```python
from build123d import *

# Parameters (mm, degrees)
F0_W     = 60
F0_H     = 20
F1_DEPTH = 5
F3_DEPTH = 2


with BuildPart() as f1:
    # F0 (on Top) → F1 (new body)
    with BuildSketch(Plane.XY):
        Rectangle(F0_W, F0_H)
    extrude(amount=F1_DEPTH)

    # F2 (on face) → F3 (cut)
    with BuildSketch(Plane.XY.offset(5)):
        with BuildLine():
            ThreePointArc((-8.9875, -4.4832849285), (-7.8815819875, -2.3618054535), (-7.5, 0))
            ThreePointArc((-7.5, 0), (-7.8815819875, 2.3618054535), (-8.9875, 4.4832849285))
            ThreePointArc((-8.9875, 4.4832849285), (-9.5314526404, 3.9326755483), (-10, 3.3166247904))
            ThreePointArc((-10, 3.3166247904), (-9.2554373535, 1.7320508076), (-9, 0))
            ThreePointArc((-9, 0), (-9.2554373535, -1.7320508076), (-10, -3.3166247904))
            ThreePointArc((-10, -3.3166247904), (-9.5314526404, -3.9326755483), (-8.9875, -4.4832849285))
        make_face()
        with BuildLine():
            ThreePointArc((-10, 3.3166247904), (-9.5314526404, 3.9326755483), (-8.9875, 4.4832849285))
            ThreePointArc((-8.9875, 4.4832849285), (-9.4660061735, 5.0621055232), (-10, 5.5901699437))
            ThreePointArc((-10, 5.5901699437), (-10.5339938265, 5.0621055232), (-11.0125, 4.4832849285))
            ThreePointArc((-11.0125, 4.4832849285), (-10.4685473596, 3.9326755483), (-10, 3.3166247904))
        make_face()
        with BuildLine():
            ThreePointArc((-10, 5.5901699437), (-9.4660061735, 5.0621055232), (-8.9875, 4.4832849285))
            ThreePointArc((-8.9875, 4.4832849285), (-5, 6), (-1.0125, 4.4832849285))
            ThreePointArc((-1.0125, 4.4832849285), (-0.5339938265, 5.0621055232), (0, 5.5901699437))
            ThreePointArc((0, 5.5901699437), (-5, 7.5), (-10, 5.5901699437))
        make_face()
        with BuildLine():
            ThreePointArc((-1.0125, -4.4832849285), (-5, -6), (-8.9875, -4.4832849285))
            ThreePointArc((-8.9875, -4.4832849285), (-9.4660061735, -5.0621055232), (-10, -5.5901699437))
            ThreePointArc((-10, -5.5901699437), (-5, -7.5), (0, -5.5901699437))
            ThreePointArc((0, -5.5901699437), (-0.5339938265, -5.0621055232), (-1.0125, -4.4832849285))
        make_face()
        with BuildLine():
            ThreePointArc((-10, -5.5901699437), (-9.4660061735, -5.0621055232), (-8.9875, -4.4832849285))
            ThreePointArc((-8.9875, -4.4832849285), (-9.5314526404, -3.9326755483), (-10, -3.3166247904))
            ThreePointArc((-10, -3.3166247904), (-10.4685473596, -3.9326755483), (-11.0125, -4.4832849285))
            ThreePointArc((-11.0125, -4.4832849285), (-10.5339938265, -5.0621055232), (-10, -5.5901699437))
        make_face()
        with BuildLine():
            ThreePointArc((-11.0125, 4.4832849285), (-10.5339938265, 5.0621055232), (-10, 5.5901699437))
            ThreePointArc((-10, 5.5901699437), (-22.5, 0), (-10, -5.5901699437))
            ThreePointArc((-10, -5.5901699437), (-10.5339938265, -5.0621055232), (-11.0125, -4.4832849285))
            ThreePointArc((-11.0125, -4.4832849285), (-21, 0), (-11.0125, 4.4832849285))
        make_face()
        with BuildLine():
            ThreePointArc((0, 5.5901699437), (-0.5339938265, 5.0621055232), (-1.0125, 4.4832849285))
            ThreePointArc((-1.0125, 4.4832849285), (-0.4685473596, 3.9326755483), (0, 3.3166247904))
            ThreePointArc((0, 3.3166247904), (0.4685473596, 3.9326755483), (1.0125, 4.4832849285))
            ThreePointArc((1.0125, 4.4832849285), (0.5339938265, 5.0621055232), (0, 5.5901699437))
        make_face()
        with BuildLine():
            ThreePointArc((0, 3.3166247904), (-0.4685473596, 3.9326755483), (-1.0125, 4.4832849285))
            ThreePointArc((-1.0125, 4.4832849285), (-2.5, 0), (-1.0125, -4.4832849285))
            ThreePointArc((-1.0125, -4.4832849285), (-0.4685473596, -3.9326755483), (0, -3.3166247904))
            ThreePointArc((0, -3.3166247904), (-1, 0), (0, 3.3166247904))
        make_face()
        with BuildLine():
            ThreePointArc((-10, -3.3166247904), (-11, 0), (-10, 3.3166247904))
            ThreePointArc((-10, 3.3166247904), (-10.4685473596, 3.9326755483), (-11.0125, 4.4832849285))
            ThreePointArc((-11.0125, 4.4832849285), (-12.5, 0), (-11.0125, -4.4832849285))
            ThreePointArc((-11.0125, -4.4832849285), (-10.4685473596, -3.9326755483), (-10, -3.3166247904))
        make_face()
        with BuildLine():
            ThreePointArc((0, -3.3166247904), (-0.4685473596, -3.9326755483), (-1.0125, -4.4832849285))
            ThreePointArc((-1.0125, -4.4832849285), (-0.5339938265, -5.0621055232), (0, -5.5901699437))
            ThreePointArc((0, -5.5901699437), (0.5339938265, -5.0621055232), (1.0125, -4.4832849285))
            ThreePointArc((1.0125, -4.4832849285), (0.4685473596, -3.9326755483), (0, -3.3166247904))
        make_face()
        with BuildLine():
            ThreePointArc((10, 5.5901699437), (5, 7.5), (0, 5.5901699437))
            ThreePointArc((0, 5.5901699437), (0.5339938265, 5.0621055232), (1.0125, 4.4832849285))
            ThreePointArc((1.0125, 4.4832849285), (5, 6), (8.9875, 4.4832849285))
            ThreePointArc((8.9875, 4.4832849285), (9.4660061735, 5.0621055232), (10, 5.5901699437))
        make_face()
        with BuildLine():
            ThreePointArc((1.0125, 4.4832849285), (0.4685473596, 3.9326755483), (0, 3.3166247904))
            ThreePointArc((0, 3.3166247904), (0.7445626465, 1.7320508076), (1, 0))
            ThreePointArc((1, 0), (0.7445626465, -1.7320508076), (0, -3.3166247904))
            ThreePointArc((0, -3.3166247904), (0.4685473596, -3.9326755483), (1.0125, -4.4832849285))
            ThreePointArc((1.0125, -4.4832849285), (2.1184180125, -2.3618054535), (2.5, 0))
            ThreePointArc((2.5, 0), (2.1184180125, 2.3618054535), (1.0125, 4.4832849285))
        make_face()
        with BuildLine():
            ThreePointArc((1.0125, -4.4832849285), (0.5339938265, -5.0621055232), (0, -5.5901699437))
            ThreePointArc((0, -5.5901699437), (5, -7.5), (10, -5.5901699437))
            ThreePointArc((10, -5.5901699437), (9.4660061735, -5.0621055232), (8.9875, -4.4832849285))
            ThreePointArc((8.9875, -4.4832849285), (5, -6), (1.0125, -4.4832849285))
        make_face()
        with BuildLine():
            ThreePointArc((22.5, 0), (18.0618621785, 6.8465319688), (10, 5.5901699437))
            ThreePointArc((10, 5.5901699437), (10.5339938265, 5.0621055232), (11.0125, 4.4832849285))
            ThreePointArc((11.0125, 4.4832849285), (17.4571324751, 5.4738012386), (21, 0))
            ThreePointArc((21, 0), (17.4571324751, -5.4738012386), (11.0125, -4.4832849285))
            ThreePointArc((11.0125, -4.4832849285), (10.5339938265, -5.0621055232), (10, -5.5901699437))
            ThreePointArc((10, -5.5901699437), (18.0618621785, -6.8465319688), (22.5, 0))
        make_face()
        with BuildLine():
            ThreePointArc((11.0125, 4.4832849285), (10.5339938265, 5.0621055232), (10, 5.5901699437))
            ThreePointArc((10, 5.5901699437), (9.4660061735, 5.0621055232), (8.9875, 4.4832849285))
            ThreePointArc((8.9875, 4.4832849285), (9.5314526404, 3.9326755483), (10, 3.3166247904))
            ThreePointArc((10, 3.3166247904), (10.4685473596, 3.9326755483), (11.0125, 4.4832849285))
        make_face()
        with BuildLine():
            ThreePointArc((8.9875, -4.4832849285), (9.4660061735, -5.0621055232), (10, -5.5901699437))
            ThreePointArc((10, -5.5901699437), (10.5339938265, -5.0621055232), (11.0125, -4.4832849285))
            ThreePointArc((11.0125, -4.4832849285), (10.4685473596, -3.9326755483), (10, -3.3166247904))
            ThreePointArc((10, -3.3166247904), (9.5314526404, -3.9326755483), (8.9875, -4.4832849285))
        make_face()
        with BuildLine():
            ThreePointArc((10, 3.3166247904), (9.5314526404, 3.9326755483), (8.9875, 4.4832849285))
            ThreePointArc((8.9875, 4.4832849285), (7.5, 0), (8.9875, -4.4832849285))
            ThreePointArc((8.9875, -4.4832849285), (9.5314526404, -3.9326755483), (10, -3.3166247904))
            ThreePointArc((10, -3.3166247904), (9, 0), (10, 3.3166247904))
        make_face()
        with BuildLine():
            ThreePointArc((12.5, 0), (12.1184180125, 2.3618054535), (11.0125, 4.4832849285))
            ThreePointArc((11.0125, 4.4832849285), (10.4685473596, 3.9326755483), (10, 3.3166247904))
            ThreePointArc((10, 3.3166247904), (10.7445626465, 1.7320508076), (11, 0))
            ThreePointArc((11, 0), (10.7445626465, -1.7320508076), (10, -3.3166247904))
            ThreePointArc((10, -3.3166247904), (10.4685473596, -3.9326755483), (11.0125, -4.4832849285))
            ThreePointArc((11.0125, -4.4832849285), (12.1184180125, -2.3618054535), (12.5, 0))
        make_face()
    extrude(amount=-F3_DEPTH, mode=Mode.SUBTRACT)


solid = f1.part
```
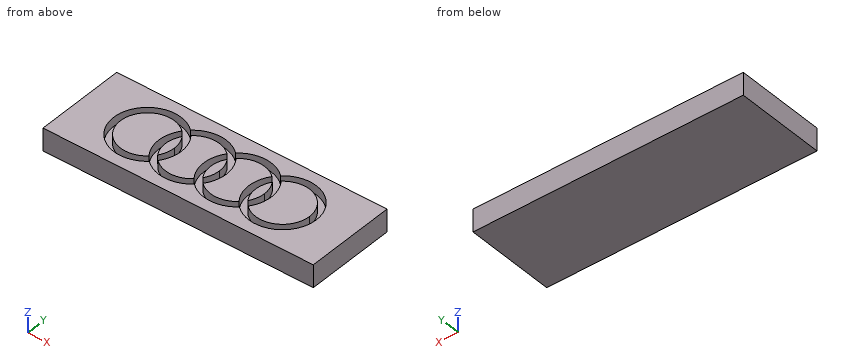
Could you check a few things on this model? Use its own coordinates, in mm. Round coordinates to 2 decimals unless told otherwise and drop trailing zeros. Write each loop counter-clockwise with the first axis right and the second up, starting at its lowest first coordinate (ties: lowest second). Pieces come first, ordered by that corner, then holes. Notation, with made-up numbers: M -37,-26.75 L 10,-26.75 A12 cw 10,-10.75 Z; hole C 74.25,76.5 d5. An arc over 180 degrees is marked long. Answer in a Markdown table with one row per item. Add a question column.
Q1. Imagine slicing it at B-B (z = 3.9). Give the number of separate pieces and of enclosed holes in the cut face, then the cut area to 3 significant figures.
Q2. Imagine slicing it at C-C (x = 14). Please give me the cut outline in (y, z), then the cut area to 3 significant figures.
Q3. If I drill on line 1 (Y direction, x = -15, z = 4.5); line 2 (X direction, y = 6.5, z = 4.4); line 3 (Z direction, x = -21, y = -1.25), over which ranges is the centre line in solid material (lowest first)? Write a range as from..to.
Q4. Imagine slicing it at A-A (x = -15). Please give me the cut outline in (y, z), then the cut area to 3 significant figures.
Q5. Will this pin go through, and if not, where does the flat tip stop? pin 1 Ø3 at (x, y) = (-8, -5) entering from -Z.
Values:
| question | item | result |
|---|---|---|
| 1 | separate pieces | 8 |
| 1 | enclosed holes | 1 |
| 1 | area | 959 mm^2 |
| 2 | outline | M -10,0 L 10,0 L 10,5 L 7.43,5 L 7.43,3 L 5.92,3 L 5.92,5 L -5.92,5 L -5.92,3 L -7.43,3 L -7.43,5 L -10,5 Z |
| 2 | area | 93.9 mm^2 |
| 3 | line 1 | -10..-7.5, -6..6, 7.5..10 |
| 3 | line 2 | -30..-18.74, -11.26..-8.74, -1.26..1.26, 8.74..11.26, 18.74..30 |
| 3 | line 3 | 0..3 |
| 4 | outline | M -10,0 L 10,0 L 10,5 L 7.5,5 L 7.5,3 L 6,3 L 6,5 L -6,5 L -6,3 L -7.5,3 L -7.5,5 L -10,5 Z |
| 4 | area | 94.0 mm^2 |
| 5 | pin 1 | z = 0 |
